Work out the finished part from the listing and answer in its coordinate system (mm). Face numbers are marked on the shaded views. Round coordinates to 2 decimals unless told otherwise and drop trailing zeros. Write each loop counter-clockwise with the first axis right and the second up, starting at its lowest first coordinate (ties: lowest second). Pieces come first, ordered by that corner, then holes. Notation, with made-up numbers: M 54.5,70.5 L 101.5,70.5 A14 ccw 101.5,82.5 Z; hole C 34,-0.75 d1. An arc over 180 degrees is marked long. Answer in a Markdown table with one row per item.
```python
from build123d import *

# Parameters (mm, degrees)
F1_DEPTH = 10
F3_D     = 1.6
F3_DEPTH = 6
F2_R     = 2.1
F4_DEPTH = 25
F5_SIZE  = 0.5


with BuildPart() as f1:
    # F0 (on Top) → F1 (new body, symmetric)
    with BuildSketch(Plane.XY):
        Polygon((-10, -3.25), (10, -3.25), (10, 3.25), (3.15, 3.25), (3.15, 0.75), (-3.15, 0.75), (-3.15, 3.25), (-10, 3.25), align=None)
    extrude(amount=F1_DEPTH, both=True)

    # F3
    with Locations(Plane.XZ.offset(3.25)):
        with Locations((0, 6.1), (0, -6.1)):
            Hole(F3_D / 2, depth=F3_DEPTH)

    # F2 (on face) → F4 (cut)
    with BuildSketch(Plane.XZ.offset(3.25)):
        Circle(F2_R)
    extrude(amount=-F4_DEPTH, mode=Mode.SUBTRACT)

    # F5
    f5_edges = [f1.edges().sort_by_distance(p)[0] for p in [
        (-3.15, 3.25, 0),
        (3.15, 3.25, 0),
    ]]
    chamfer(f5_edges, length=F5_SIZE)


solid = f1.part
```
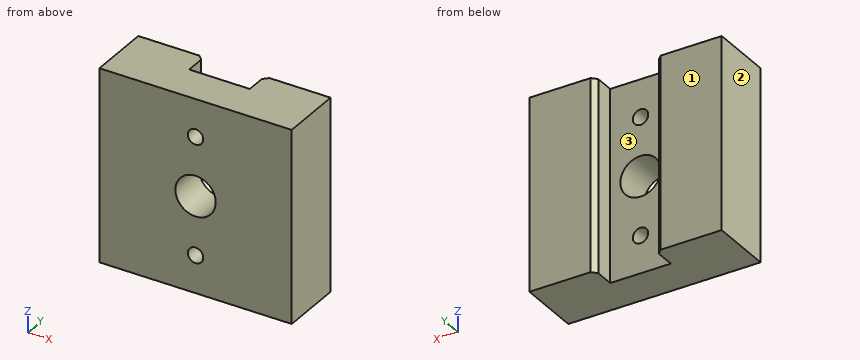
1. Determine the mould class of the marked faces 1, 2 and 3 for opening direction X: released by +X, released by -X, zero draft, split by the parting line, or undercut.
Calculated:
| item | result |
|---|---|
| face 1 | zero draft |
| face 2 | released by -X |
| face 3 | undercut |
2. Consider line 1 along Z through (x, y) = (0, -1.8); line 2 along X through (y, z) = (1.5, 3.75); line 3 along X through (y, z) = (-0.75, 6). Determine where each line is inside the solid, lowest interval first. Write a range as from..to.
Calculated:
| item | result |
|---|---|
| line 1 | z = -10..-6.9, -5.3..-2.1, 2.1..5.3, 6.9..10 |
| line 2 | x = -10..-3.15, 3.15..10 |
| line 3 | x = -10..-0.79, 0.79..10 |
3. Given pin 1 (5 mm diameter, centred on x = -0.5, z = -4.5, fed in from +Y), flat-ended and moving along its own axis, determine where the tip first touches the part or whether it passes through.
Calculated:
| item | result |
|---|---|
| pin 1 | stops at y = 0.75 |
4. The part is cut by section C-C (y = 0.5). Determine the outline of the cut face in (x, z), plus the area to 3 significant figures.
Calculated:
| item | result |
|---|---|
| outline | M -10,-10 L 10,-10 L 10,10 L -10,10 Z; hole C 0,0 d4.2; hole C 0,-6.1 d1.6; hole C 0,6.1 d1.6 |
| area | 382 mm² |
5. The part is cut by section B-B (x = 0). Determine the outline of the cut face in (y, z).
Calculated:
| item | result |
|---|---|
| outline | M -3.25,-10 L 0.75,-10 L 0.75,-6.9 L -3.25,-6.9 Z; M -3.25,-5.3 L 0.75,-5.3 L 0.75,-2.1 L -3.25,-2.1 Z; M -3.25,2.1 L 0.75,2.1 L 0.75,5.3 L -3.25,5.3 Z; M -3.25,6.9 L 0.75,6.9 L 0.75,10 L -3.25,10 Z |
6. The part is cut by section D-D (z = 6.1). Determine the outline of the cut face in (x, y), plus the area to 3 significant figures.
Calculated:
| item | result |
|---|---|
| outline | M -10,-3.25 L -0.8,-3.25 L -0.8,0.75 L -3.15,0.75 L -3.15,2.75 L -3.65,3.25 L -10,3.25 Z; M 0.8,-3.25 L 10,-3.25 L 10,3.25 L 3.65,3.25 L 3.15,2.75 L 3.15,0.75 L 0.8,0.75 Z |
| area | 108 mm² |
7. The part is cut by section A-A (y = 2). Determine the outline of the cut face in (x, z).
Calculated:
| item | result |
|---|---|
| outline | M -10,-10 L -3.15,-10 L -3.15,10 L -10,10 Z; M 3.15,-10 L 10,-10 L 10,10 L 3.15,10 Z |
